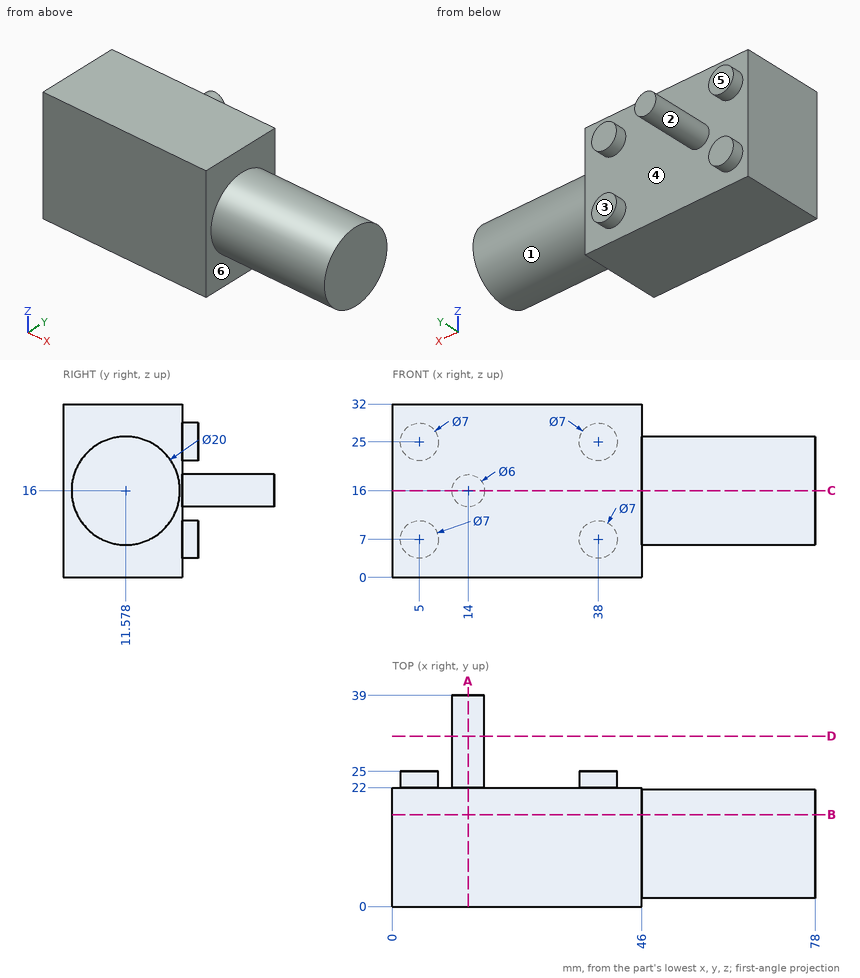
Check sheet for the drawn part. Datum: minimum x, y, z corner. Units: mm. A direction names the side the tool comes from. Round coordinates to 2 decimals unless told otherwise and drop trailing zeros. Loops run counter-clockwise (first coordinate to the right, second up) from the corner with the lowest first, then second, coordinate; pieces in that order, holes last.
Item 1: Cross-section at C-C on z = 16. Record the boundary of the cut face in (x, y), then the cut area to 3 significant figures.
Item 2: Thickness scan on line 1 (Y direction, x = 7.5, z = 4); line 2 (Y direction, x = 4, z = 4); line 3 (X direction, y = 7, z = 2.5). Record the ranges inside material, lowest first.
Item 3: Cross-section at B-B on y = 17. Record the boundary of the cut face in (x, z).
Item 4: Gauge pin test, flat ends, axial feed: pin 1 (7.5 mm diameter, centred on x = 6.5, z = 24.5, fed in from +Y); pin 2 (1.5 mm diameter, centred on x = 32.5, y = 22.5, fed in from +Z); pin 3 (6 mm diameter, centred on x = 31.5, z = 21.5, fed in from +Y); pin 4 (5 mm diameter, centred on x = 61.5, y = 9, fed in from +Z). Record the tip position at first contact, or that the pin passes through.
Item 5: Mould release check, pull along X, two halves, no side actions. Record for the marked faces 4, 5 and 6: pulls with the +X half, pulls with the -X half, needs draft (parallel to the pull), parting line crosses it, or undercut.
Item 6: Cross-section at A-A on x = 14. Record the boundary of the cut face in (y, z).
Item 7: Access from +Z, -Z, +X, -X, +Y, -Y to the whole of each face (thin tool, end or side, straight path). Record for the marked faces 1, 2 and 3.
Item 8: Cross-section at D-D on y = 31.5. Record the boundary of the cut face in (x, z).
Answer sheet:
1. outline: (0, 0) - (46, 0) - (46, 1.58) - (78, 1.58) - (78, 21.58) - (46, 21.58) - (46, 22) - (17, 22) - (17, 39) - (11, 39) - (11, 22) - (0, 22) - close
1. area: 1,750 mm2
2. line 1: y = 0 to 22
2. line 2: y = 0 to 25
2. line 3: x = 0 to 46
3. outline: (0, 0) - (46, 0) - (46, 7.6) - (78, 7.6) - (78, 24.4) - (46, 24.4) - (46, 32) - (0, 32) - close
4. pin 1: stops at y = 25
4. pin 2: stops at z = 32
4. pin 3: stops at y = 22
4. pin 4: stops at z = 26
5. face 4: undercut
5. face 5: needs draft
5. face 6: pulls with the +X half
6. outline: (0, 0) - (22, 0) - (22, 13) - (39, 13) - (39, 19) - (22, 19) - (22, 32) - (0, 32) - close
7. face 1: +X
7. face 2: +Y
7. face 3: +Z, -Z, +X, -X, +Y
8. outline: circle Ø6 at (14, 16)
